Geometry: final body of the model. Coordinates: model frame, mm. A direction names the side the tool comes from. Coordinates: 2 decimals unless noted, no trailing zeros. Loops run counter-clockwise (first coordinate to the right, second up) from the corner with the lowest first, then second, coordinate; pieces in that order, holes last. Notation, with made-up numbers: (61, -39.75) - (96, -39.75) arc R27 cw to (96, -17.75) - close; hole circle Ø6 at (22.25, 51). An arc over 180 degrees is marked (long way). Write each question's results on one line, items separated by ' | '. Start each with the question number.
from build123d import *
from build123d.topology import SkipClean

# Parameters (mm, degrees)
ESBO_O1_W                  = 14
ESBO_O1_H                  = 20
ESBO_O1_R                  = 1.25
RESSALTO_EXTRUS_O1_DEPTH   = 14
ESBO_O6_R                  = 2.75
CORTE_EXTRUS_O3_DEPTH      = 10
CORTE_EXTRUS_O5_DEPTH      = 10
CORTE_EXTRUS_O5_DEPTH_BACK = 10
ESBO_O3_R                  = 1.25
ESBO_O8_R                  = 3.05
CORTE_EXTRUS_O6_DEPTH      = 10
ESBO_O9_OUTSIDE_W          = 21.628
ESBO_O9_OUTSIDE_H          = 21.628
ESBO_O9_OUTSIDE_R          = 7
CORTE_EXTRUS_O7_DEPTH      = 26.396850332
RESSALTO_EXTRUS_O2_START   = -6.122497316
RESSALTO_EXTRUS_O2_DEPTH   = 2.244994532
RESSALTO_EXTRUS_O3_DEPTH   = 10
ESBO_O13_R                 = 1.3
CORTE_EXTRUS_O8_DEPTH      = 16
RESSALTO_EXTRUS_O4_DEPTH   = 10
ESBO_O15_R                 = 1.3
CORTE_EXTRUS_O9_DEPTH      = 7
ESBO_O16_R                 = 7.5
ESBO_O16_R_2               = 7
RESSALTO_EXTRUS_O5_DEPTH   = 3
FILETE2_R                  = 2
FILETE3_R                  = 2
RESSALTO_EXTRUS_O6_START   = 10
RESSALTO_EXTRUS_O6_DEPTH   = 10
CORTE_EXTRUS_O11_DEPTH     = 10
CORTE_EXTRUS_O12_DEPTH     = 10
RESSALTO_EXTRUS_O8_DEPTH   = 10
RESSALTO_EXTRUS_O9_DEPTH   = 10
RESSALTO_EXTRUS_O10_DEPTH  = 10
ESBO_O26_R                 = 7
ESBO_O26_R_2               = 3.45
RESSALTO_EXTRUS_O11_DEPTH  = 20
FILETE4_R                  = 1.5
FILETE5_R                  = 1.5
ESBO_O27_W                 = 5.34202784
ESBO_O27_H                 = 3.157877353
RESSALTO_EXTRUS_O12_DEPTH  = 8


# Read off the part's stored shape, not the designer's step: Ressalto-extrusão2
with BuildPart() as part:
    # Esboço1 → Ressalto-extrusão1 (new body)
    with BuildSketch(Plane(origin=(0, 0, 0), x_dir=(1, 0, 0), z_dir=(0, 1, 0))):
        Rectangle(ESBO_O1_W, ESBO_O1_H)
        with Locations(Location((0, 5, 0), (0, 0, 270))):
            Circle(ESBO_O1_R, mode=Mode.SUBTRACT)
    extrude(amount=RESSALTO_EXTRUS_O1_DEPTH)

    # Esboço6 → Corte-extrusão3 (cut)
    with BuildSketch(Plane(origin=(0, 0, -10), x_dir=(-1, 0, 0), z_dir=(0, 0, -1))):
        with Locations((0, 7)):
            Circle(ESBO_O6_R)
    extrude(amount=-CORTE_EXTRUS_O3_DEPTH, mode=Mode.SUBTRACT)

    # Esboço3 → Corte-extrusão5 (cut, two sides: drawn at the far end of the back side and taken through both)
    with BuildSketch(Plane(origin=(0, 0, 0), x_dir=(1, 0, 0), z_dir=(0, 1, 0)).offset(-CORTE_EXTRUS_O5_DEPTH_BACK)):
        with Locations(Location((0, -5, 0), (0, 0, 270))):
            Circle(ESBO_O3_R)
    extrude(amount=CORTE_EXTRUS_O5_DEPTH + CORTE_EXTRUS_O5_DEPTH_BACK, mode=Mode.SUBTRACT)

    # Esboço8 → Corte-extrusão6 (cut)
    with BuildSketch(Plane.XY.offset(10)):
        with Locations((0, 7)):
            Circle(ESBO_O8_R)
    extrude(amount=-CORTE_EXTRUS_O6_DEPTH, mode=Mode.SUBTRACT)

    # Esboço9 outside → Corte-extrusão7 (cut, through all)
    with BuildSketch(Plane.XY.offset(10)):
        with Locations((0, 7)):
            Rectangle(ESBO_O9_OUTSIDE_W, ESBO_O9_OUTSIDE_H)
        with Locations((0, 7)):
            Circle(ESBO_O9_OUTSIDE_R, mode=Mode.SUBTRACT)
    extrude(amount=-CORTE_EXTRUS_O7_DEPTH, mode=Mode.SUBTRACT)

    # Ressalto-extrusão2 outline → Ressalto-extrusão2 (add)
    with SkipClean():  # the faces are left unmerged after this step: merging them gives an invalid solid
        with BuildSketch(Plane.XY.offset(10).offset(RESSALTO_EXTRUS_O2_START)):
            with BuildLine():
                ThreePointArc((0.55, 10), (2.343074903, 8.952562419), (3.05, 7))
                Line((3.05, 7), (7, 7))
                ThreePointArc((7, 7), (0, 14), (-7, 7))
                Line((-7, 7), (-3.05, 7))
                ThreePointArc((-3.05, 7), (-2.343074903, 8.952562419), (-0.55, 10))
                ThreePointArc((-0.55, 10), (0, 10.05), (0.55, 10))
            make_face()
        extrude(amount=RESSALTO_EXTRUS_O2_DEPTH)

    # Esboço11 → Ressalto-extrusão3 (add)
    with SkipClean():  # the faces are left unmerged after this step: merging them gives an invalid solid
        with BuildSketch(Plane(origin=(0, 0, -10), x_dir=(-1, 0, 0), z_dir=(0, 0, -1))):
            with BuildLine():
                Line((2.079062289, 5.2), (-2.079062289, 5.2))
                ThreePointArc((-2.079062289, 5.2), (0, 4.25), (2.079062289, 5.2))
            make_face()
            with BuildLine():
                ThreePointArc((2.079062289, 8.8), (0, 9.75), (-2.079062289, 8.8))
                Line((-2.079062289, 8.8), (2.079062289, 8.8))
            make_face()
        extrude(amount=-RESSALTO_EXTRUS_O3_DEPTH)

    # Esboço13 → Corte-extrusão8 (cut)
    with BuildSketch(Plane(origin=(0, 0, 0), x_dir=(1, 0, 0), z_dir=(0, 1, 0))):
        with Locations(Location((0, 5, 0), (0, 0, 90))):
            Circle(ESBO_O13_R)
    extrude(amount=CORTE_EXTRUS_O8_DEPTH, mode=Mode.SUBTRACT)

    # Esboço14 → Ressalto-extrusão4 (add)
    with BuildSketch(Plane.XY.offset(10)):
        with BuildLine():
            Line((0, 3.95), (0, 4.95))
            Line((0, 4.95), (-2.258317958, 4.95))
            ThreePointArc((-2.258317958, 4.95), (-1.234908904, 4.211183047), (0, 3.95))
        make_face()
        with BuildLine():
            Line((2.258317958, 4.95), (0, 4.95))
            Line((0, 4.95), (0, 3.95))
            ThreePointArc((0, 3.95), (1.234908904, 4.211183047), (2.258317958, 4.95))
        make_face()
    extrude(amount=-RESSALTO_EXTRUS_O4_DEPTH)

    # Esboço15 → Corte-extrusão9 (cut)
    with BuildSketch(Plane(origin=(0, 0, 0), x_dir=(1, 0, 0), z_dir=(0, 1, 0))):
        with Locations(Location((0, -5, 0), (0, 0, 90))):
            Circle(ESBO_O15_R)
    extrude(amount=CORTE_EXTRUS_O9_DEPTH, mode=Mode.SUBTRACT)

    # Esboço16 → Ressalto-extrusão5 (add, symmetric)
    with BuildSketch(Plane.XY):
        with Locations((0, 7)):
            Circle(ESBO_O16_R)
        with Locations((0, 7)):
            Circle(ESBO_O16_R_2, mode=Mode.SUBTRACT)
    extrude(amount=RESSALTO_EXTRUS_O5_DEPTH, both=True)

    # Filete2
    # the kernel refuses this fillet: 2 mm, written as the material it takes off along each edge
    with BuildSketch(Plane(origin=(0, 7, 3), x_dir=(1, 0, 0), z_dir=(0, -1, 0))) as filete2_piece_1:
        with BuildLine():
            CenterArc((5.5, -1.322875656), FILETE2_R, 0, 41.409622109)
            Line((7, 0), (7.03, 0.026457513))
            ThreePointArc((7.03, 0.026457513), (7.25, 0.04), (7.5, 0.04))
            Line((7.5, 0.04), (7.54, 0))
            Line((7.54, 0), (7.54, -1.322875656))
            Line((7.54, -1.322875656), (7.5, -1.322875656))
        make_face()
    revolve(axis=Axis((0, 7, 3), (0, 0, 1)), mode=Mode.SUBTRACT)

    # Filete3
    # the kernel refuses this fillet: 2 mm, written as the material it takes off along each edge
    with BuildSketch(Plane(origin=(0, 7, -3), x_dir=(1, 0, 0), z_dir=(0, -1, 0))) as filete3_piece_1:
        with BuildLine():
            CenterArc((5.5, 1.322875656), FILETE3_R, 318.590377891, 41.409622109)
            Line((7.5, 1.322875656), (7.54, 1.322875656))
            Line((7.54, 1.322875656), (7.54, 0))
            Line((7.54, 0), (7.5, -0.04))
            ThreePointArc((7.5, -0.04), (7.25, -0.04), (7.03, -0.026457513))
            Line((7.03, -0.026457513), (7, 0))
        make_face()
    revolve(axis=Axis((0, 7, -3), (0, 0, 1)), mode=Mode.SUBTRACT)

    # Esboço18 → Ressalto-extrusão6 (add)
    with BuildSketch(Plane.XY.offset(RESSALTO_EXTRUS_O6_START)):
        with BuildLine():
            Line((2.46221445, 5.2), (2.079062289, 5.2))
            Line((2.079062289, 5.2), (-2.079062289, 5.2))
            Line((-2.079062289, 5.2), (-2.46221445, 5.2))
            ThreePointArc((-2.46221445, 5.2), (-2.363573895, 5.072302294), (-2.258317958, 4.95))
            Line((-2.258317958, 4.95), (2.258317958, 4.95))
            ThreePointArc((2.258317958, 4.95), (2.363573895, 5.072302294), (2.46221445, 5.2))
        make_face()
    extrude(amount=-RESSALTO_EXTRUS_O6_DEPTH)

    # Esboço19 → Corte-extrusão11 (cut)
    with BuildSketch(Plane.XY.offset(10)):
        with BuildLine():
            ThreePointArc((-2.46221445, 5.2), (0, 10.05), (2.46221445, 5.2))
            Line((2.46221445, 5.2), (3.059820256, 5.2))
            ThreePointArc((3.059820256, 5.2), (0, 10.55), (-3.059820256, 5.2))
            Line((-3.059820256, 5.2), (-2.46221445, 5.2))
        make_face()
    extrude(amount=-CORTE_EXTRUS_O11_DEPTH, mode=Mode.SUBTRACT)

    # Esboço20 → Corte-extrusão12 (cut)
    with BuildSketch(Plane(origin=(0, 0, -10), x_dir=(-1, 0, 0), z_dir=(0, 0, -1))):
        with BuildLine():
            Line((-2.494493937, 4.2), (2.494493937, 4.2))
            ThreePointArc((2.494493937, 4.2), (3.75, 7), (2.494493937, 9.8))
            Line((2.494493937, 9.8), (-2.494493937, 9.8))
            ThreePointArc((-2.494493937, 9.8), (-3.75, 7), (-2.494493937, 4.2))
        make_face()
        with BuildLine():
            Line((-2.079062289, 8.8), (2.079062289, 8.8))
            ThreePointArc((2.079062289, 8.8), (2.75, 7), (2.079062289, 5.2))
            Line((2.079062289, 5.2), (-2.079062289, 5.2))
            ThreePointArc((-2.079062289, 5.2), (-2.75, 7), (-2.079062289, 8.8))
        make_face(mode=Mode.SUBTRACT)
    extrude(amount=-CORTE_EXTRUS_O12_DEPTH, mode=Mode.SUBTRACT)

    # Esboço23 → Ressalto-extrusão8 (add)
    with BuildSketch(Plane(origin=(0, 0, -10), x_dir=(-1, 0, 0), z_dir=(0, 0, -1))):
        with BuildLine():
            Line((-2.494493937, 4.2), (2.494493937, 4.2))
            ThreePointArc((2.494493937, 4.2), (3.75, 7), (2.494493937, 9.8))
            Line((2.494493937, 9.8), (-2.494493937, 9.8))
            ThreePointArc((-2.494493937, 9.8), (-3.75, 7), (-2.494493937, 4.2))
        make_face()
        with BuildLine():
            Line((-2.369493617, 9.48), (2.369493617, 9.48))
            ThreePointArc((2.369493617, 9.48), (3.43, 7), (2.369493617, 4.52))
            Line((2.369493617, 4.52), (-2.369493617, 4.52))
            ThreePointArc((-2.369493617, 4.52), (-3.43, 7), (-2.369493617, 9.48))
        make_face(mode=Mode.SUBTRACT)
    extrude(amount=-RESSALTO_EXTRUS_O8_DEPTH)

    # Esboço24 → Ressalto-extrusão9 (add)
    with BuildSketch(Plane.XY.offset(10)):
        with BuildLine():
            Line((3.059820256, 5.2), (-3.059820256, 5.2))
            ThreePointArc((-3.059820256, 5.2), (0, 10.55), (3.059820256, 5.2))
        make_face()
        with BuildLine():
            Line((2.972793299, 5.35), (-2.972793299, 5.35))
            ThreePointArc((-2.972793299, 5.35), (0, 10.4), (2.972793299, 5.35))
        make_face(mode=Mode.SUBTRACT)
    extrude(amount=-RESSALTO_EXTRUS_O9_DEPTH)

    # Esboço25 → Ressalto-extrusão10 (add)
    with BuildSketch(Plane(origin=(0, 0, -10), x_dir=(-1, 0, 0), z_dir=(0, 0, -1))):
        with BuildLine():
            Line((2.369493617, 9.48), (-2.369493617, 9.48))
            ThreePointArc((-2.369493617, 9.48), (-3.43, 7), (-2.369493617, 4.52))
            Line((-2.369493617, 4.52), (2.369493617, 4.52))
            ThreePointArc((2.369493617, 4.52), (3.43, 7), (2.369493617, 9.48))
        make_face()
        with BuildLine():
            Line((2.245996438, 9.18), (-2.245996438, 9.18))
            ThreePointArc((-2.245996438, 9.18), (-3.13, 7), (-2.245996438, 4.82))
            Line((-2.245996438, 4.82), (2.245996438, 4.82))
            ThreePointArc((2.245996438, 4.82), (3.13, 7), (2.245996438, 9.18))
        make_face(mode=Mode.SUBTRACT)
    extrude(amount=-RESSALTO_EXTRUS_O10_DEPTH)

    # Esboço26 → Ressalto-extrusão11 (add)
    with BuildSketch(Plane.XY.offset(10)):
        with Locations((0, 7)):
            Circle(ESBO_O26_R)
        with Locations((0, 7)):
            Circle(ESBO_O26_R_2, mode=Mode.SUBTRACT)
    extrude(amount=-RESSALTO_EXTRUS_O11_DEPTH)

    # Filete4
    filete4_edges = [part.edges().sort_by_distance(p)[0] for p in [
        (-7, 7, -10),
    ]]
    fillet(filete4_edges, radius=FILETE4_R)

    # Filete5
    filete5_edges = [part.edges().sort_by_distance(p)[0] for p in [
        (-7, 7, 10),
    ]]
    fillet(filete5_edges, radius=FILETE5_R)

    # Esboço27 → Ressalto-extrusão12 (add)
    with BuildSketch(Plane.XY.offset(10)):
        with Locations((0, 3.771061324)):
            Rectangle(ESBO_O27_W, ESBO_O27_H)
    extrude(amount=-RESSALTO_EXTRUS_O12_DEPTH)


solid = part.part
1) Pull-direction query (Z, two-part tool) for faces 1 (the flat face through (0.1, 4.6, -10)), 2 (the flat face through (0, 9.4, 0)), 3 (the cylindrical face through (-3.13, 6.97, -5.07)), 4 (the cylindrical face through (-0.02, 3.55, -4.98)); classes: released by +Z, released by -Z, zero draft, split by the parting line, or undercut.
2) Section query C-C on z = -5. Output: boundary loops of the cut face in (x, y).
3) Section query B-B on x = 0. Count the separate pieces of the cut face and the enclosed holes in it, and give its area (3 significant figures).
4) Access query for faces 5 (the flat face through (0, 4.2, -5)), 6 (the flat face through (0, 4.82, -5)), 7 (the flat face through (0, 9.18, -5)). Directions: +Z, -Z, +X, -X, +Y, -Y. A direction counts if a zero-diameter tool reaches every point of the face in a straight line with its end or side. Return the directions, or none.
5) Material intervals for line 1 (Z direction, x = 0.25, y = 9.5); line 2 (X direction, y = 7, z = 5.75); line 3 (X direction, y = 3.85, z = -5), sorted ascending. Write a range as [from, to].
6) Pin query (flat end, axial travel): pin 1 Ø1.5 at (x, y) = (-5, 11) entering from +Z; pin 2 Ø2 at (x, z) = (0.5, -5) entering from +Y; pin 3 Ø1.5 at (x, y) = (-1, 7.5) entering from +Z; pin 4 Ø4 at (y, z) = (9.5, -7.5) entering from +X. Return the tip coordinate at first contact, or that it passes through.
7) Section query D-D on z = -7.75. Output: boundary loops of the cut face in (x, y), and give its area (3 significant figures).
8) Section query A-A on y = 7. Output: boundary loops of the cut face in (x, z), and give its area (3 significant figures).
Returned:
1) face 1: released by -Z | face 2: released by +Z | face 3: zero draft | face 4: undercut
2) outline: circle Ø14 at (0, 7); hole (-2.25, 4.82) - (2.25, 4.82) arc R3.13 ccw to (2.25, 9.18) - (-2.25, 9.18) arc R3.13 ccw to start; hole (-1.3, 3.8) arc R3.45 ccw to (1.3, 3.8) - (1.3, 4.2) - (-1.3, 4.2) - close; hole (-1.3, 9.8) - (1.3, 9.8) - (1.3, 10.2) arc R3.45 ccw to (-1.3, 10.2) - close
3) separate pieces: 2 | enclosed holes: 2 | area: 186 mm²
4) face 5: none | face 6: -Z | face 7: +Z, -Z
5) line 1: z = [-10, 0] | line 2: x = [-7, -3.4], [3.4, 7] | line 3: x = [-6.25, -1.3], [1.3, 6.25]
6) pin 1: stops at z = 9.99 | pin 2: stops at y = 14 | pin 3: passes through | pin 4: stops at x = 6.98
7) outline: circle Ø14 at (0, 7); hole (-2.25, 4.82) - (2.25, 4.82) arc R3.13 ccw to (2.25, 9.18) - (-2.25, 9.18) arc R3.13 ccw to start | area: 129 mm²
8) outline: (-7.5, -1.68) arc R2 ccw to (-7, -3) - (-7, -8.5) arc R1.5 ccw to (-5.5, -10) - (-3.13, -10) - (-3.13, 0) - (-3.4, 0) - (-3.4, 10) - (-5.5, 10) arc R1.5 ccw to (-7, 8.5) - (-7, 3) arc R2 ccw to (-7.5, 1.68) - close; (3.13, -10) - (5.5, -10) arc R1.5 ccw to (7, -8.5) - (7, -3) arc R2 ccw to (7.5, -1.68) - (7.5, 1.68) arc R2 ccw to (7, 3) - (7, 8.5) arc R1.5 ccw to (5.5, 10) - (3.4, 10) - (3.4, 0) - (3.13, 0) - close | area: 153 mm²
